Here's how the part is built. I have some questions about the finished solid (model axes, mm). A direction names the side the tool comes from. Coordinates: 2 decimals unless noted, no trailing zeros. Write each loop counter-clockwise with the first axis right and the second up, starting at its lowest first coordinate (ties: lowest second). Pieces come first, ordered by that corner, then holes. Notation, with made-up numbers: (24, -28.5) -> (36, -28.5) arc R19 cw to (36, -3.5) -> close; hole circle Ø1 at (-0.75, 16). An arc over 180 degrees is marked (long way). Use CSV: the item, a comma, the result in double quotes. Start each with the question number.
```python
from build123d import *

# Parameters (mm, degrees)
SKETCH1_R             = 4.95
BOSS_EXTRUDE1_DEPTH   = 2
BOSS_EXTRUDE1_2_DEPTH = 2
BOSS_EXTRUDE1_3_DEPTH = 2
BOSS_EXTRUDE1_4_DEPTH = 2
SKETCH2_W             = 39
SKETCH2_H             = 103.4
BOSS_EXTRUDE2_DEPTH   = 2
SKETCH3_W             = 6
SKETCH3_H             = 2
CUT_EXTRUDE1_DEPTH    = 88.767775977
CUT_EXTRUDE2_DEPTH    = 88.767775977


with BuildPart() as part:
    # Sketch1 → Boss-Extrude1 (new body)
    with BuildSketch(Plane(origin=(0, 0, 0), x_dir=(1, 0, 0), z_dir=(0, 1, 0))):
        with Locations(Location((-15.2, 60, 0), (0, 0, 270))):
            Circle(SKETCH1_R)
    extrude(amount=BOSS_EXTRUDE1_DEPTH)



with BuildPart() as body_2:
    # Sketch1 → Boss-Extrude1 2 (new body)
    with BuildSketch(Plane(origin=(0, 0, 0), x_dir=(1, 0, 0), z_dir=(0, 1, 0))):
        with Locations(Location((15.2, 60, 0), (0, 0, 270))):
            Circle(SKETCH1_R)
    extrude(amount=BOSS_EXTRUDE1_2_DEPTH)


with BuildPart() as body_3:
    # Sketch1 → Boss-Extrude1 3 (new body)
    with BuildSketch(Plane(origin=(0, 0, 0), x_dir=(1, 0, 0), z_dir=(0, 1, 0))):
        with Locations(Location((15.2, 0, 0), (0, 0, 270))):
            Circle(SKETCH1_R)
    extrude(amount=BOSS_EXTRUDE1_3_DEPTH)


with BuildPart() as body_4:
    # Sketch1 → Boss-Extrude1 4 (new body)
    with BuildSketch(Plane(origin=(0, 0, 0), x_dir=(1, 0, 0), z_dir=(0, 1, 0))):
        with Locations(Location((-15.2, 0, 0), (0, 0, 270))):
            Circle(SKETCH1_R)
    extrude(amount=BOSS_EXTRUDE1_4_DEPTH)


with BuildPart() as part_1:
    add(part.part)

    add(body_2.part)  # Boss-Extrude2 merges body 2

    add(body_3.part)  # Boss-Extrude2 merges body 3

    add(body_4.part)  # Boss-Extrude2 merges body 4
    # Sketch2 → Boss-Extrude2 (add)
    with BuildSketch(Plane(origin=(0, 2, 0), x_dir=(1, 0, 0), z_dir=(0, 1, 0))):
        with Locations((0, 33.7)):
            Rectangle(SKETCH2_W, SKETCH2_H)
    extrude(amount=-BOSS_EXTRUDE2_DEPTH)

    # Sketch3 → Cut-Extrude1 (cut, through all)
    with BuildSketch(Plane(origin=(0, 2, 0), x_dir=(1, 0, 0), z_dir=(0, 1, 0))):
        with Locations((0, 84.4)):
            Rectangle(SKETCH3_W, SKETCH3_H)
    extrude(amount=-CUT_EXTRUDE1_DEPTH, mode=Mode.SUBTRACT)

    # Sketch5 → Cut-Extrude2 (cut, through all)
    with BuildSketch(Plane.XZ):
        with BuildLine():
            Line((18.5, -62.170829335), (18.5, -57.829170665))
            ThreePointArc((18.5, -57.829170665), (19.15, -60), (18.5, -62.170829335))
        make_face()
        with BuildLine():
            Line((18.5, -2.170829335), (18.5, 2.170829335))
            ThreePointArc((18.5, 2.170829335), (19.15, 0), (18.5, -2.170829335))
        make_face()
        with BuildLine():
            Line((-18.5, -2.170829335), (-18.5, 2.170829335))
            ThreePointArc((-18.5, 2.170829335), (-19.15, 0), (-18.5, -2.170829335))
        make_face()
        with BuildLine():
            Line((-18.5, -62.170829335), (-18.5, -57.829170665))
            ThreePointArc((-18.5, -57.829170665), (-19.15, -60), (-18.5, -62.170829335))
        make_face()
    extrude(amount=-CUT_EXTRUDE2_DEPTH, mode=Mode.SUBTRACT)


solid = part_1.part
```
Item 1: Which directions (+Z, -Z, +X, -X, +Y, -Y) give clear straight access to the entire face, cutting with the end or side of a thin tool? Please do faces 5 (the flat face through (19.5, 1, -74)), 6 (the flat face through (19.5, 1, 10)), 7 (the flat face through (0, 1, -83.4)).
Item 2: I'm going to push flat-ended pins straight in: pin 1 (0.6 mm diameter, centred on y = 1.5, z = -69.5, fed in from +X); pin 2 (0.6 mm diameter, centred on y = 1.5, z = 12.5, fed in from -X); pin 3 (0.6 mm diameter, centred on y = 1, z = 0.5, fed in from -X). Where does each tip first touch, or does it pass through?
Item 3: If I drill on line 1 along X through (y, z) = (0.2, -3); line 2 along Z through (x, y) = (2.5, 1.6), over which ranges is the centre line in solid material (lowest first)?
Item 4: I want a section at C-C on z = -73.5. Please give me the cut outline in (x, y), then the cut area to 3 significant figures.
Item 5: Thinking about a two-plate mould opening in Z: for faces 1 (the flat face through (-3, 1, -84)), 2 (the cylindrical face through (-20.15, 0.99, -60.04)), 3 (the flat face through (-11, 1, -85.4)), 4 (the flat face through (-18.5, 1, -60)), which applies, +Z half, -Z half, draft (parallel to the pull), parting line (faces both ways), or undercut?
Item 6: I want a section at B-B on x = -2. Please give me the cut outline in (y, z), then the cut area to 3 significant figures.
Item 7: I want a section at A-A on y = 0.75. Please give me the cut outline in (x, z), then the cut area to 3 significant figures.
Geometry says:
1,face 5,"-Z, +X, +Y, -Y"
1,face 6,"+Z, +X, +Y, -Y"
1,face 7,"-Z, +Y, -Y"
2,pin 1,"x = 19.5"
2,pin 2,"x = -19.5"
2,pin 3,"x = -20.15"
3,line 1,"-19.5 to 19.5"
3,line 2,"-83.4 to 18"
4,outline,"(-19.5, 0) -> (19.5, 0) -> (19.5, 2) -> (-19.5, 2) -> close"
4,area,"78.0 mm2"
5,face 1,"draft"
5,face 2,"undercut"
5,face 3,"-Z half"
5,face 4,"undercut"
6,outline,"(0, -83.4) -> (2, -83.4) -> (2, 18) -> (0, 18) -> close"
6,area,"203 mm2"
7,outline,"(-19.5, -85.4) -> (-3, -85.4) -> (-3, -83.4) -> (3, -83.4) -> (3, -85.4) -> (19.5, -85.4) -> (19.5, -62.45) arc R4.95 ccw to (19.5, -57.55) -> (19.5, -2.45) arc R4.95 ccw to (19.5, 2.45) -> (19.5, 18) -> (-19.5, 18) -> (-19.5, 2.45) arc R4.95 ccw to (-19.5, -2.45) -> (-19.5, -57.55) arc R4.95 ccw to (-19.5, -62.45) -> close; hole (-18.5, -62.17) -> (-18.5, -57.83) arc R3.95 ccw to start; hole (-18.5, -2.17) -> (-18.5, 2.17) arc R3.95 ccw to start; hole (18.5, -62.17) arc R3.95 ccw to (18.5, -57.83) -> close; hole (18.5, -2.17) arc R3.95 ccw to (18.5, 2.17) -> close"
7,area,"4,020 mm2"
